Source: CAD feature listing. Evaluate the final solid. Frame: model axes, mm. Give positions to 0.01 mm unless a question says otherwise; leave off trailing zeros. Write each loop counter-clockwise with the first axis right and the second up, starting at its lowest first coordinate (ties: lowest second). Pieces come first, ordered by that corner, then holes. Notation, with made-up numbers: (54.25, 7) -> (66.25, 7) arc R21 ccw to (66.25, 46) -> close; hole circle Ø3 at (36, -14.75). An arc over 180 degrees is marked (long way). Use one line per item in the form item = value. Start each with the question number.
(1) Material intervals for line 1 along Y through (x, z) = (0, -327.5); line 2 along X through (y, z) = (0, 325.25); line 3 along Y through (x, z) = (-1.5, -228), sorted ascending. Write a range as from..to.
(2) Cut plane A-A, the plane z = 79.5. Output: boundary loops of the cut face in (x, y).
(3) First-contact query: P1, Ø2, axis at y = -5, z = -167.5, coming from the -X side; P2, Ø1, axis at x = 1, z = 175, coming from the +Y side; P3, Ø4.5, axis at x = 0, y = 0, coming from the -Z side. Flat tips, straight axial feed; report the tip coordinate or a pass-through.
Autodesk Inventor part; units mm, degrees
ref_plane "YZ Plane" through (0, 0, 0) normal (1, 0, 0) x (0, 1, 0)
ref_plane "XZ Plane" through (0, 0, 0) normal (0, 1, 0) x (-1, 0, 0)
ref_plane "XY Plane" through (0, 0, 0) normal (0, 0, 1) x (1, 0, 0)
sketch "Sketch1" plane through (0, 0, 0) normal (0, 0, 1) x (1, 0, 0)
  line L0 (0, 7.3323) -> (6.35, 3.6662)
  line L1 (6.35, 3.6662) -> (6.35, -3.6662)
  line L2 (6.35, -3.6662) -> (0, -7.3323)
  line L3 (0, -7.3323) -> (-6.35, -3.6662)
  line L4 (-6.35, -3.6662) -> (-6.35, 3.6662)
  line L5 (-6.35, 3.6662) -> (0, 7.3323)
  point P0 (0, 0)
  point P1 (0, 0)
  dimension "d1" = 12.7
extrude "Extrusion1" add sketch "Sketch1" along normal mid plane 668.1267
sketch "Sketch2" plane through (0, 0, 334.0633) normal (0, 0, 1) x (1, 0, 0)
  point P0 (0, 0)
hole "Hole1" at (0, 0, 334.0633) direction (0, 0, -1) diameter 4.9784 depth 19.05 tip angle 118
mirror "Mirror1" about plane through (0, 0, 0) normal (0, 0, 1) of "Hole1"
properties part number "0.5_Jack_Shaft" material "Aluminum, 6061-T6"
Geometry says:
q1.line_1 = -7.33..-2.49, 2.49..7.33
q1.line_2 = -6.35..-2.49, 2.49..6.35
q1.line_3 = -6.47..6.47
q2.outline = (-6.35, -3.67) -> (0, -7.33) -> (6.35, -3.67) -> (6.35, 3.67) -> (0, 7.33) -> (-6.35, 3.67) -> close
q3.P1 = -5.77
q3.P2 = 7.04
q3.P3 = -314.87
